Here's how the part is built. I have some questions about the finished solid (model axes, mm). Face numbers are marked on the shaded views. A direction names the side the tool comes from. Give positions to 0.01 mm unless a question says otherwise; leave off trailing zeros. Write each loop counter-clockwise with the first axis right and the second up, starting at its lowest first coordinate (ties: lowest second). Pieces come first, ordered by that corner, then holes. Notation, with made-up numbers: (25, 61.25) - (55, 61.25) arc R18 ccw to (55, 85.25) - close; hole circle Ø4 at (2.25, -13). An arc over 180 degrees is marked (long way). Use a Markdown table: item, result.
Autodesk Inventor part; units mm, degrees
ref_plane "YZ Plane" through (0, 0, 0) normal (1, 0, 0) x (0, 1, 0)
ref_plane "XZ Plane" through (0, 0, 0) normal (0, 1, 0) x (-1, 0, 0)
ref_plane "XY Plane" through (0, 0, 0) normal (0, 0, 1) x (1, 0, 0)
sketch "Sketch1" plane through (0, 0, 0) normal (0, 1, 0) x (-1, 0, 0)
  line L0 (20.0643, 8.1272) -> (19.9344, -8.4408)
  line L1 (19.9344, -8.4408) -> (8.1272, -20.0643)
  line L2 (8.1272, -20.0643) -> (-8.4408, -19.9344)
  line L3 (-8.4408, -19.9344) -> (-20.0643, -8.1272)
  line L4 (-20.0643, -8.1272) -> (-19.9344, 8.4408)
  line L5 (-19.9344, 8.4408) -> (-8.1272, 20.0643)
  line L6 (-8.1272, 20.0643) -> (8.4408, 19.9344)
  line L7 (8.4408, 19.9344) -> (20.0643, 8.1272)
  point P0 (0, 0)
  point P1 (0, 0)
  dimension "d0" = 20
  dimension "d1" = 16.568
extrude "Extrusion1" add sketch "Sketch1" along normal blind 2
sketch "Sketch2" plane through (0, 2, 0) normal (0, 1, 0) x (1, 0, 0)
  line L0 (15.0642, 6.0559) -> (14.9342, -6.3698)
  line L1 (14.9342, -6.3698) -> (6.0559, -15.0642)
  line L2 (6.0559, -15.0642) -> (-6.3698, -14.9342)
  line L3 (-6.3698, -14.9342) -> (-15.0642, -6.0559)
  line L4 (-15.0642, -6.0559) -> (-14.9342, 6.3698)
  line L5 (-14.9342, 6.3698) -> (-6.0559, 15.0642)
  line L6 (-6.0559, 15.0642) -> (6.3698, 14.9342)
  line L7 (6.3698, 14.9342) -> (15.0642, 6.0559)
  point P0 (0, 0)
  point P1 (0, 0)
  dimension "d4" = 15
  dimension "d5" = 12.4257
extrude "Extrusion2" add sketch "Sketch2" along normal blind 2
properties part number "oktagonUnten"
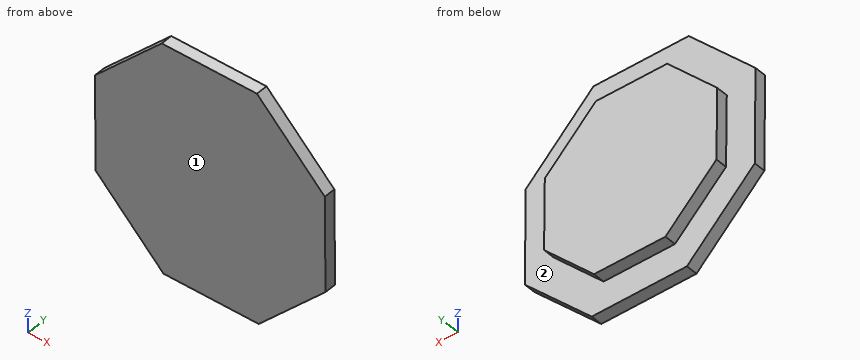
Item 1: I need wall thicknesses on line 1 along X through (y, z) = (1, -7); line 2 along Y through (x, z) = (16, 5); line 3 along Z through (x, y) = (4.5, 0.25). Which ranges of each line are inside material? Lowest first, please. Write a range as [from, to].
Values:
| item | result |
|---|---|
| line 1 | x = [-19.95, 20.06] |
| line 2 | y = [0, 2] |
| line 3 | z = [-19.97, 20.04] |
Item 2: If we section it at C-C, the plane x = 16.5: Write out the boundary of the cut face in (y, z), plus the area to 3 significant figures.
Values:
| item | result |
|---|---|
| outline | (0, -11.75) - (2, -11.75) - (2, 11.82) - (0, 11.82) - close |
| area | 47.1 mm2 |
Item 3: If we section it at B-B, the plane z = -14: Write out the boundary of the cut face in (x, y).
Values:
| item | result |
|---|---|
| outline | (-14.29, 0) - (14.28, 0) - (14.28, 2) - (7.28, 2) - (7.28, 4) - (-7.14, 4) - (-7.14, 2) - (-14.29, 2) - close |
Item 4: For the marked faces 1 and 2, which set-ups out of +Z, -Z, +X, -X, +Y, -Y let a thin tool reach every point of the face, with its end or its side?
Values:
| item | result |
|---|---|
| face 1 | +Z, -Z, +X, -X, -Y |
| face 2 | +Y |
Item 5: Will these pins go through, and if not, where does the flat tip stop? pin 1 Ø2 at (y, z) = (1, 0) entering from -X; pin 2 Ø1 at (x, y) = (14, 1) entering from -Z; pin 3 Ø1 at (x, y) = (-14.5, 3.5) entering from +Z.
Values:
| item | result |
|---|---|
| pin 1 | stops at x = -20.01 |
| pin 2 | stops at z = -14.8 |
| pin 3 | stops at z = 7.14 |
Item 6: If we section it at A-A, the plane y = 1.5: Write out the boundary of the cut face in (x, z).
Values:
| item | result |
|---|---|
| outline | (-20.06, 8.13) - (-19.93, -8.44) - (-8.13, -20.06) - (8.44, -19.93) - (20.06, -8.13) - (19.93, 8.44) - (8.13, 20.06) - (-8.44, 19.93) - close |
